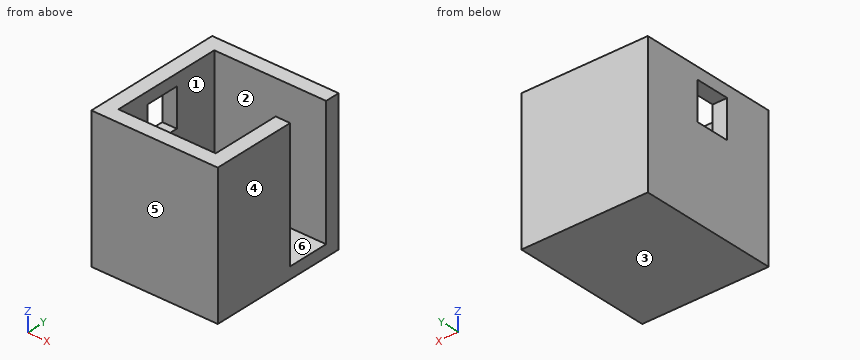
```python
from build123d import *

# Parameters (mm, degrees)
F2_DEPTH  = 20
F3_W      = 217
F3_H      = 242
F3_W_2    = 167
F3_H_2    = 192
F4_DEPTH  = 240
F5_W      = 48
F5_H      = 72
F6_DEPTH  = 250
F7_W      = 79
F7_H      = 85
F8_DEPTH  = 25
F10_DEPTH = 25


with BuildPart() as f2:
    # F1 (on face) → F2 (new body)
    with BuildSketch(Plane.XY):
        Polygon((-497, -215), (-497, -231), (-497, -293), (-497, -407), (-330, -407), (-330, -287), (-330, -215), align=None)
    extrude(amount=F2_DEPTH)

    # F3 (on face) → F4 (join)
    with BuildSketch(Plane.XY):
        with Locations((-413.5, -311)):
            Rectangle(F3_W, F3_H)
        with Locations((-413.5, -311)):
            Rectangle(F3_W_2, F3_H_2, mode=Mode.SUBTRACT)
    extrude(amount=F4_DEPTH)

    # F5 (on face) → F6 (cut)
    with BuildSketch(Plane.XY.offset(20)):
        with Locations((-306, -251)):
            Rectangle(F5_W, F5_H)
    extrude(amount=F6_DEPTH, mode=Mode.SUBTRACT)

    # F7 (on face) → F8 (cut)
    with BuildSketch(Plane.YZ.offset(-497)):
        with Locations((-309.5, 177.5)):
            Rectangle(F7_W, F7_H)
    extrude(amount=-F8_DEPTH, mode=Mode.SUBTRACT)

    # F9 (on face) → F10 (join, through all)
    with BuildSketch(Plane.YZ.offset(-497)):
        Polygon((-270, 135), (-270, 220), (-290, 220), (-290, 155), (-349, 155), (-349, 135), align=None)
    extrude(amount=-F10_DEPTH)


solid = f2.part
```
Part model, mm, in its own coordinate system. Face numbers are marked on the shaded views. A direction names the side the tool comes from. Give positions to 0.01 mm unless a question says otherwise; leave off trailing zeros. Write each loop counter-clockwise with the first axis right and the second up, starting at its lowest first coordinate (ties: lowest second). Pieces come first, ordered by that corner, then holes. Notation, with made-up numbers: (48, 38.5) -> (71, 38.5) arc R18 cw to (71, 59.5) -> close; hole circle Ø4 at (17, 82.5). An arc over 180 degrees is marked (long way). Put each result on its own line as item: value. Start each with the question number.
Item 1: Cut at C-C (x = -410). List the corners of the cut face in (y, z), then the cut area to 3 significant figures.
Item 2: Cut at B-B (y = -318). List the corners of the cut face in (x, z), then the cut area to 3 significant figures.
Item 3: Which spindle directions (+Z, -Z, +X, -X, +Y, -Y) get a long thin tool onto all of the face, cutting with end or side? Do the marked faces 1, 2 and 3. Say none if no direction does.
Item 4: Cut at A-A (z = 213). List the corners of the cut face in (x, y), then the cut area to 3 significant figures.
Item 5: Wall check: L1, parallel to X at y = -304.5, z = 137.5; L2, parallel to Y at x = -317.5, z = 33; L3, parallel to Y at x = -337.5, z = 58. Give the ranges that are in metal, low to high. Write a range as [from, to].
Item 6: Cut at D-D (z = 135). List the corners of the cut face in (x, y).
Item 7: Pull direction Y, two halves, no side cores. Call the marked faces 4, 5 and 6: pulls with the +Y half, pulls with the -Y half, needs draft (parallel to the pull), parting line crosses it, or undercut.
Item 8: Pin check, flat tips, straight feed: pin 1 Ø1 at (x, y) = (-454, -395) entering from -Z; pin 2 Ø1.5 at (x, y) = (-450.5, -232) entering from +Z. Stop position of each tip, or through.
Answer list:
1. outline: (-432, 0) -> (-190, 0) -> (-190, 240) -> (-215, 240) -> (-215, 20) -> (-407, 20) -> (-407, 240) -> (-432, 240) -> close
1. area: 15,800 mm2
2. outline: (-522, 0) -> (-305, 0) -> (-305, 240) -> (-330, 240) -> (-330, 20) -> (-497, 20) -> (-497, 155) -> (-522, 155) -> close; (-522, 220) -> (-497, 220) -> (-497, 240) -> (-522, 240) -> close
2. area: 13,700 mm2
3. face 1: +Z
3. face 2: +Z, +X
3. face 3: -Z, +X, -X, +Y, -Y
4. outline: (-522, -432) -> (-305, -432) -> (-305, -287) -> (-330, -287) -> (-330, -407) -> (-497, -407) -> (-497, -349) -> (-522, -349) -> close; (-522, -290) -> (-497, -290) -> (-497, -215) -> (-305, -215) -> (-305, -190) -> (-522, -190) -> close
4. area: 17,200 mm2
5. L1: x = [-522, -497], [-330, -305]
5. L2: y = [-432, -287], [-215, -190]
5. L3: y = [-432, -407], [-215, -190]
6. outline: (-522, -432) -> (-305, -432) -> (-305, -287) -> (-330, -287) -> (-330, -407) -> (-497, -407) -> (-497, -215) -> (-305, -215) -> (-305, -190) -> (-522, -190) -> close
7. face 4: needs draft
7. face 5: pulls with the -Y half
7. face 6: undercut
8. pin 1: stops at z = 0
8. pin 2: stops at z = 20
